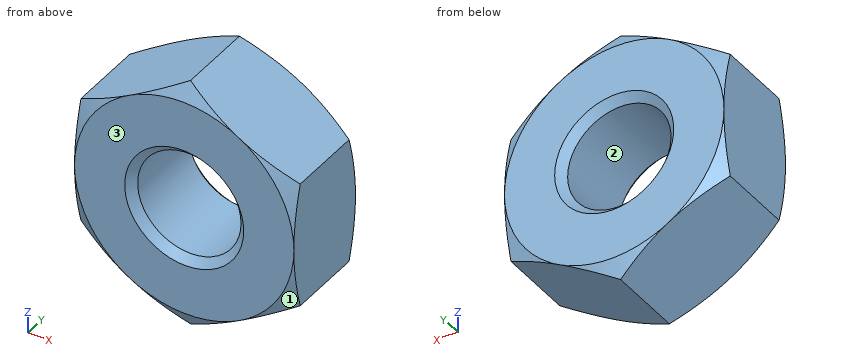
from build123d import *

# Parameters (mm, degrees)
BOSS_EXTRUDE1_DEPTH     = 1.5
SKETCH2_OUTSIDE_W       = 19.534
SKETCH2_OUTSIDE_H       = 20.616
SKETCH2_OUTSIDE_R       = 3.5
CUT_EXTRUDE1_DEPTH      = 2.4
CUT_EXTRUDE1_DRAFT      = -60
MIRROR1_COPY_1_SKETCH_W = 19.534
MIRROR1_COPY_1_SKETCH_H = 20.616
MIRROR1_COPY_1_SKETCH_R = 3.5
MIRROR1_COPY_1_DEPTH    = 2.4
MIRROR1_COPY_1_DRAFT    = -60
TAPPED_HOLE1_D          = 3.3
CHAMFER1_SIZE           = 0.25


with BuildPart() as part:
    # Sketch1 → Boss-Extrude1 (new, symmetric)
    with BuildSketch(Plane(origin=(0, 0, 0), x_dir=(1, 0, 0), z_dir=(0, 1, 0))):
        Polygon((3.5, -2.020725942), (3.5, 2.020725942), (0, 4.041451884), (-3.5, 2.020725942), (-3.5, -2.020725942), (0, -4.041451884), align=None)
    extrude(amount=BOSS_EXTRUDE1_DEPTH, both=True)


with BuildPart() as cut_extrude1_tool:
    # Sketch2 outside → Cut-Extrude1 (with draft: the straight prism first)
    with BuildSketch(Plane(origin=(0, 1.5, 0), x_dir=(1, 0, 0), z_dir=(0, 1, 0))):
        Rectangle(SKETCH2_OUTSIDE_W, SKETCH2_OUTSIDE_H)
        Circle(SKETCH2_OUTSIDE_R, mode=Mode.SUBTRACT)
    extrude(amount=-CUT_EXTRUDE1_DEPTH)
    # Cut-Extrude1: the draft: its side faces are tilted about the plane it starts from
    cut_extrude1_sides = [cut_extrude1_tool.faces().sort_by_distance(p)[0] for p in [
        (0, 0.3, 10.308),
        (9.767, 0.3, 0),
        (0, 0.3, -10.308),
        (-9.767, 0.3, 0),
        (-3.5, 0.3, 0),
    ]]
    draft(cut_extrude1_sides, Plane(origin=(0, 1.5, 0), x_dir=(1, 0, 0), z_dir=(0, 1, 0)), CUT_EXTRUDE1_DRAFT)


with BuildPart() as part_1:
    add(part.part)

    # Cut-Extrude1: cut by cut_extrude1_tool
    add(cut_extrude1_tool.part, mode=Mode.SUBTRACT)


with BuildPart() as mirror1_copy_1_tool:
    # Mirror1 copy 1 sketch → Mirror1 copy 1 (with draft: the straight prism first)
    with BuildSketch(Plane.XZ.offset(1.5)):
        Rectangle(MIRROR1_COPY_1_SKETCH_W, MIRROR1_COPY_1_SKETCH_H)
        Circle(MIRROR1_COPY_1_SKETCH_R, mode=Mode.SUBTRACT)
    extrude(amount=-MIRROR1_COPY_1_DEPTH)
    # Mirror1 copy 1: the draft: its side faces are tilted about the plane it starts from
    mirror1_copy_1_sides = [mirror1_copy_1_tool.faces().sort_by_distance(p)[0] for p in [
        (0, -0.3, 10.308),
        (9.767, -0.3, 0),
        (0, -0.3, -10.308),
        (-9.767, -0.3, 0),
        (-3.5, -0.3, 0),
    ]]
    draft(mirror1_copy_1_sides, Plane.XZ.offset(1.5), MIRROR1_COPY_1_DRAFT)


with BuildPart() as part_2:
    add(part_1.part)

    # Mirror1 copy 1: cut by mirror1_copy_1_tool
    add(mirror1_copy_1_tool.part, mode=Mode.SUBTRACT)

    # Tapped Hole1 (through all)
    with Locations(Plane(origin=(0, -1.5, 0), x_dir=(-1, 0, 0), z_dir=(0, -1, 0))):
        with Locations((0, 0)):
            Hole(TAPPED_HOLE1_D / 2)

    # Chamfer1
    chamfer1_edges = [part_2.edges().sort_by_distance(p)[0] for p in [
        (-1.65, -1.5, 0),
        (-1.65, 1.5, 0),
    ]]
    chamfer(chamfer1_edges, length=CHAMFER1_SIZE)


solid = part_2.part
The model under review builds one solid part; all positions refer to its coordinate system, in mm. Face numbers are marked on the shaded views. Give positions to 0.01 mm unless a question says otherwise; leave off trailing zeros. Write each loop counter-clockwise with the first axis right and the second up, starting at its lowest first coordinate (ties: lowest second). Pieces come first, ordered by that corner, then holes. Notation, with made-up numbers: M 13.25,2 L 63.25,2 A9 cw 63.25,12 Z; hole C 46,36.5 d9. An arc over 180 degrees is marked long. One line per question, with ' | ' between items. Start each with the question number.
Item 1: Wall thickness on line 1 (X direction, y = 0, z = 0); line 2 (Z direction, x = 0.25, y = 1.35); line 3 (Z direction, x = 0.5, y = -0.15): over which ranges is each line inside the solid? List them lowest first. Write a range as from..to.
Item 2: We need section A-A on y = 0.3. Write out the cut boundary in (x, z), plus the area to 3 significant figures.
Item 3: For pin 1 (3 mm diameter, centred on x = 0, z = 0, fed in from -Y), flat-tipped, find the tip position at first contact; note if it passes through.
Item 4: Draft analysis for pull direction X (two halves, no side actions). For the marked faces 1, 2 and 3, state which applies: released by +X, released by -X, zero draft, split by the parting line, or undercut.
Results found:
1) line 1: x = -3.5..-1.65, 1.65..3.5 | line 2: z = -3.75..-1.73, 1.73..3.75 | line 3: z = -3.75..-1.57, 1.57..3.75
2) outline: M -3.5,-2.02 L 0,-4.04 L 3.5,-2.02 L 3.5,2.02 L 0,4.04 L -3.5,2.02 Z; hole C 0,0 d3.3 | area: 33.9 mm2
3) pin 1: passes through
4) face 1: released by +X | face 2: undercut | face 3: zero draft
